Study the drawing (mm; zero at the part's minimum x, y, z) and answer. A direction names the side the tool comes from. Round coordinates to 2 decimals unless told otherwise and drop trailing zeros. Write each loop counter-clockwise with the first axis right and the second up, starting at its lowest first coordinate (ties: lowest second). Pieces come first, ordered by that corner, then holes. Notation, with made-up numbers: (-20, 13) - (-1, 13) arc R10 cw to (-1, 18) - close; hole circle Ø3 at (3.5, 10). An arc over 180 degrees is marked (long way). Use one line per item in the form item = value. Start each with the question number.
1) The part is cut by section A-A, the plane x = 12. Give the vertices of the cut face in (y, z), plus the area to 3 significant figures.
2) The part is cut by section C-C, the plane y = 24.25. Count the separate pieces of the cut face and the enclosed holes in it.
3) Consider line 1 along Z through (x, y) = (12, 18.5); line 2 along Z through (x, y) = (12, 4.4); line 3 along Z through (x, y) = (12, 17.45). Determine where each line is inside the solid, lowest interval first. Write a range as from..to.
4) The part is cut by section B-B, the plane z = 7.5. Give the vertices of the cut face in (x, y) (1 decimal).
5) For the marked faces 1 and 2, determine the directions among +Z, -Z, +X, -X, +Y, -Y from which every point of the face is accessible in a straight line to the end or side of a thin tool.
6) Each of these flat-tipped pins is pushed along its axis until it touches: pin 1 (3 mm diameter, centred on y = 9.5, z = 11.5, fed in from +X); pin 2 (3 mm diameter, centred on x = 11.5, z = 12, fed in from -Y); pin 3 (5 mm diameter, centred on x = 13, y = 23, fed in from -Z). Where does it stop, or does it pass through?
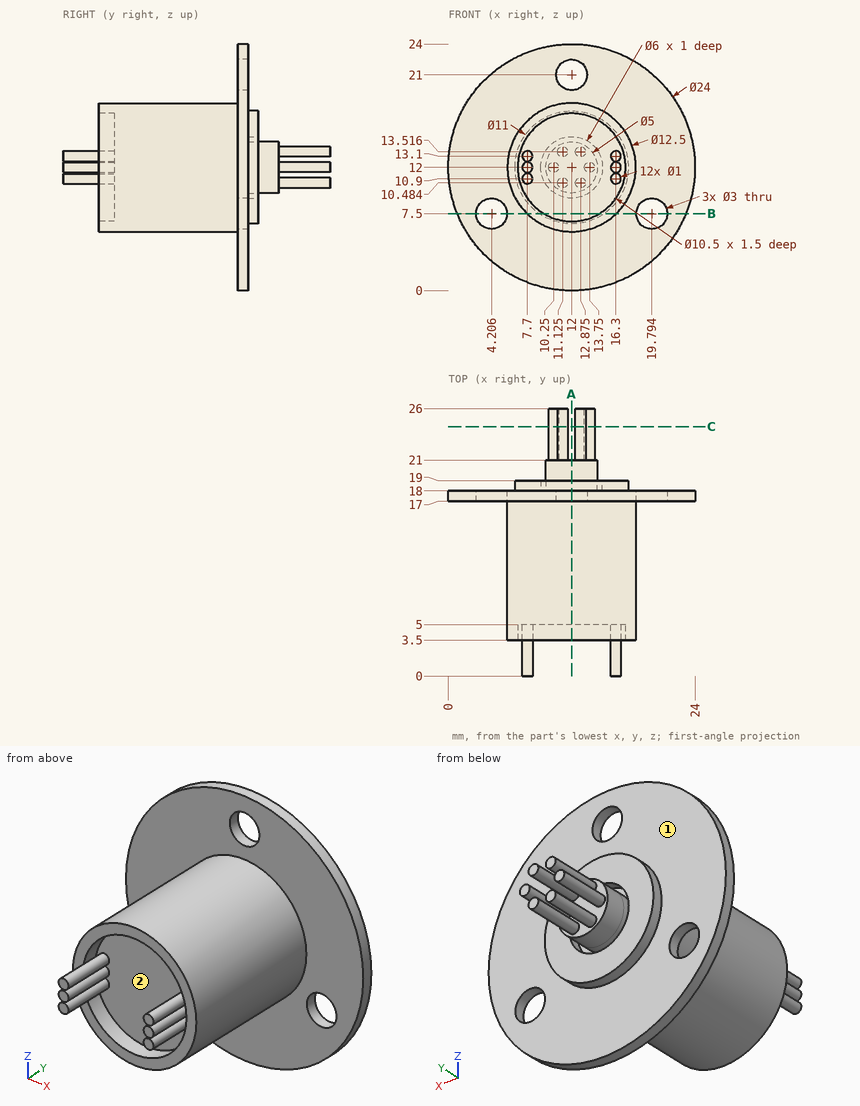
Geometry results:
q1.outline = (3.5, 5.75) - (17, 5.75) - (17, 0) - (18, 0) - (18, 6.5) - (19, 6.5) - (19, 9) - (18, 9) - (18, 9.5) - (21, 9.5) - (21, 14.5) - (18, 14.5) - (18, 15) - (19, 15) - (19, 17.5) - (18, 17.5) - (18, 19.5) - (17, 19.5) - (17, 18.25) - (3.5, 18.25) - (3.5, 17.25) - (5, 17.25) - (5, 6.75) - (3.5, 6.75) - close; (17, 22.5) - (18, 22.5) - (18, 24) - (17, 24) - close
q1.area = 194 mm2
q2.separate_pieces = 6
q2.enclosed_holes = 0
q3.line_1 = 6.5..9, 9.5..14.5, 15..17.5
q3.line_2 = 5.75..6.75, 17.25..18.25
q3.line_3 = 0..19.5, 22.5..24
q4.outline = (0.9, 17) - (2.7, 17) - (2.7, 18) - (0.9, 18) - close; (5.7, 17) - (7.7, 17) - (7.7, 3.5) - (9.3, 3.5) - (9.3, 5) - (14.7, 5) - (14.7, 3.5) - (16.3, 3.5) - (16.3, 17) - (18.3, 17) - (18.3, 18) - (15.2, 18) - (15.2, 19) - (8.8, 19) - (8.8, 18) - (5.7, 18) - close; (21.3, 17) - (23.1, 17) - (23.1, 18) - (21.3, 18) - close
q5.face_1 = +Y
q5.face_2 = -Y
q6.pin_1 = 18.25
q6.pin_2 = 5
q6.pin_3 = 9.5
